Geometry check sheet. Reference: drawing and pictorial views, mm from the part's lowest x, y, z. A direction names the side the tool comes from. Round coordinates to 2 decimals unless told otherwise and drop trailing zeros. Write each loop counter-clockwise with the first axis right and the second up, starting at its lowest first coordinate (ties: lowest second). Pieces come first, ordered by that corner, then holes. Notation, with made-up numbers: (41, 35) - (97, 35) arc R8 ccw to (97, 40) - close; hole circle Ø11 at (63, 43). An arc over 180 degrees is marked (long way). Use one line per item in the form item = value. Start each with the question number.
1) Section check B-B (x = 16.75). Record the boundary of the cut face in (y, z).
2) Section check C-C (y = 3.5). Record the boundary of the cut face in (x, z).
3) Gauge pin test, flat ends, axial feed: P1, Ø1.5, axis at x = 8.5, z = 25.5, coming from the -Y side; P2, Ø3, axis at x = 5.62, y = 6.8, coming from the +Z side; P3, Ø2.5, axis at x = 4.12, z = 21, coming from the +Y side; P4, Ø1.6, axis at x = 25.38, z = 21, coming from the +Y side. Record the tip position at first contact, or that the pin passes through.
4) Set-up check for the marked faces 1 and 2: record each of +Z, -Z, +X, -X, +Y, -Y from which the full face is reachable in a straight line by a thin tool's end or side.
5) Section check A-A (x = 23.5). Record the boundary of the cut face in (y, z) (1 decimal), then the cut area to 3 significant figures.
6) Scan line: probe 1 along Z at (x, y) = (9, 4.75). Record every from-to range of solid material in increasing order.
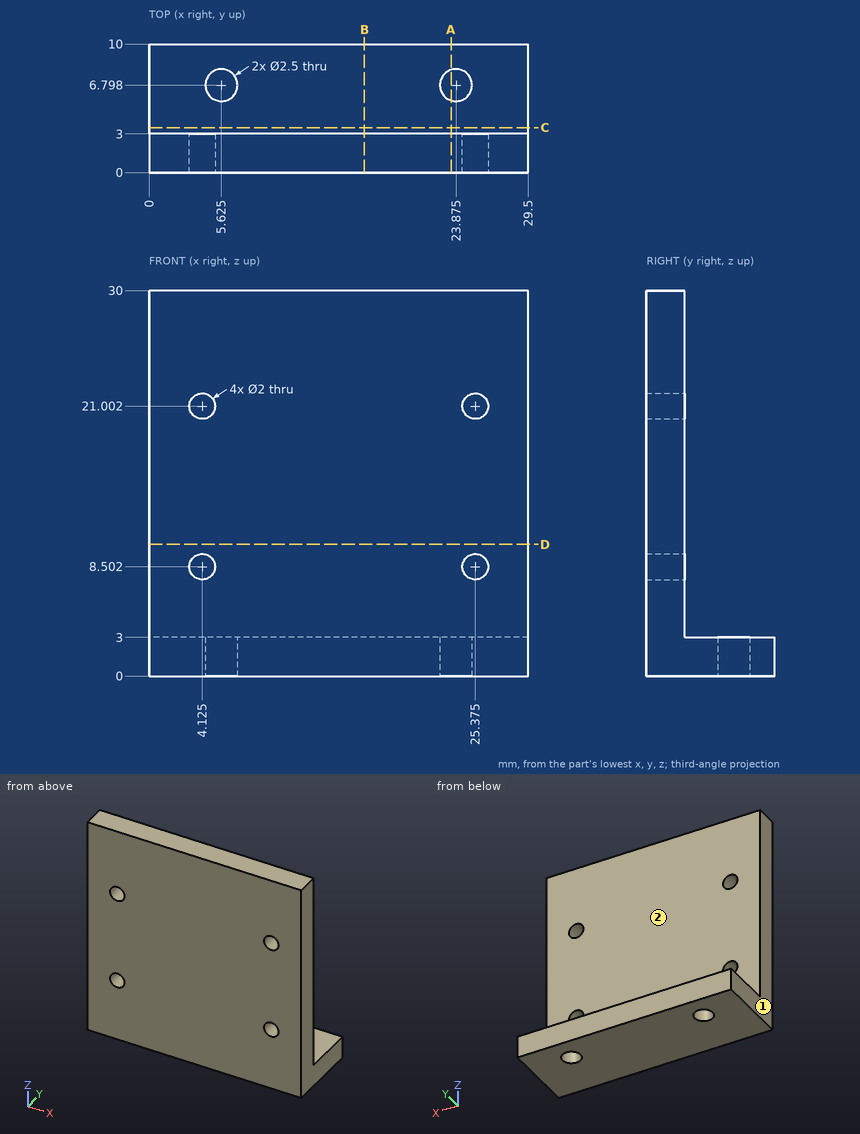
Results are:
q1.outline = (0, 0) - (10, 0) - (10, 3) - (3, 3) - (3, 30) - (0, 30) - close
q2.outline = (0, 0) - (29.5, 0) - (29.5, 3) - (0, 3) - close
q3.P1 = 0
q3.P2 = 3
q3.P3 = 3
q3.P4 = through
q4.face_1 = +Z, -Z, -X, +Y, -Y
q4.face_2 = +Z, +X, -X, +Y
q5.outline = (0, 0) - (5.6, 0) - (5.6, 3) - (3, 3) - (3, 30) - (0, 30) - close; (8, 0) - (10, 0) - (10, 3) - (8, 3) - close
q5.area = 104 mm²
q6.probe_1 = 0 to 3
